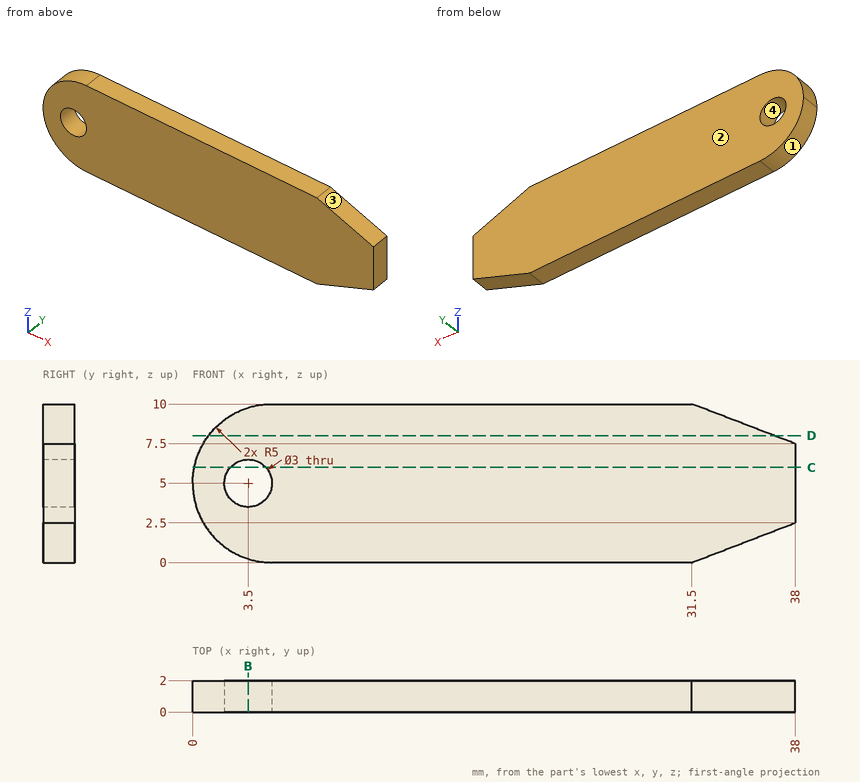
The figure shows three views and two pictorial views of one solid part (mm, origin at its lowest corner). Answer the questions. Give positions to 0.01 mm unless a question says otherwise; leave off trailing zeros. Write each loop counter-clockwise with the first axis right and the second up, starting at its lowest first coordinate (ties: lowest second). Pieces come first, ordered by that corner, then holes. Notation, with made-up numbers: M 5.5,-17 L 43.5,-17 A19 ccw 43.5,4 Z; hole C 75.5,-31.5 d8. An arc over 180 degrees is marked long. One line per item, written item: value. Start each with the question number.
(1) Find the intervals of material crossed by line 1 (X direction, y = 1.1, z = 5); line 2 (X direction, y = 0.2, z = 7); line 3 (Z direction, x = 34.5, y = 1.35), in increasing order.
(2) Find section B-B (x = 3.5). Determine the outline of the cut face in (y, z), plus the area to 3 significant figures.
(3) Determine the mould class of the marked faces 1, 2, 3 and 4 for opening direction Z: pulls with the +Z half, pulls with the -Z half, needs draft (parallel to the pull), parting line crosses it, or undercut.
(4) Find section D-D (z = 8). Determine the outline of the cut face in (x, y).
(5) Find section C-C (z = 6). Determine the outline of the cut face in (x, y), plus the area to 3 significant figures.
Results below:
1. line 1: x = 0 to 2, 5 to 38
1. line 2: x = 0.42 to 38
1. line 3: z = 1.15 to 8.85
2. outline: M 0,0.23 L 2,0.23 L 2,3.5 L 0,3.5 Z; M 0,6.5 L 2,6.5 L 2,9.77 L 0,9.77 Z
2. area: 13.1 mm^2
3. face 1: pulls with the -Z half
3. face 2: needs draft
3. face 3: pulls with the +Z half
3. face 4: undercut
4. outline: M 1,0 L 36.7,0 L 36.7,2 L 1,2 Z
5. outline: M 0.1,0 L 2.38,0 L 2.38,2 L 0.1,2 Z; M 4.62,0 L 38,0 L 38,2 L 4.62,2 Z
5. area: 71.3 mm^2
